```python
from build123d import *

# Parameters (mm, degrees)
SKIZZE1_W                                            = 50
SKIZZE1_H                                            = 60
AUFSATZ_LINEAR_AUSTRAGEN1_DEPTH                      = 5
FORMSENKUNG_F_R_M5_LINSENSENKSCHRAUBE_MI_D           = 5.5
FORMSENKUNG_F_R_M5_LINSENSENKSCHRAUBE_MI_DEPTH       = 20
FORMSENKUNG_F_R_M5_LINSENSENKSCHRAUBE_MI_CSINK_D     = 11
FORMSENKUNG_F_R_M5_LINSENSENKSCHRAUBE_MI_CSINK_ANGLE = 90
FORMSENKUNG_F_R_M5_LINSENSENKSCHRAUBE_MI_TIP         = 1.652366702
KERNLOCH_F_R_M4_GEWINDE1_D                           = 3.3
KERNLOCH_F_R_M5_GEWINDE1_D                           = 4.2
VERRUNDUNG1_R                                        = 3


with BuildPart() as part:
    # Skizze1 → Aufsatz-Linear austragen1 (new body)
    with BuildSketch(Plane.XY):
        with Locations((0, 30)):
            Rectangle(SKIZZE1_W, SKIZZE1_H)
    extrude(amount=-AUFSATZ_LINEAR_AUSTRAGEN1_DEPTH)

    # Formsenkung für M5 Linsensenkschraube mit Schlitz1
    with Locations(Plane.XY):
        with Locations((-16, 10), (16, 10)):
            CounterSinkHole(FORMSENKUNG_F_R_M5_LINSENSENKSCHRAUBE_MI_D / 2, FORMSENKUNG_F_R_M5_LINSENSENKSCHRAUBE_MI_CSINK_D / 2, depth=FORMSENKUNG_F_R_M5_LINSENSENKSCHRAUBE_MI_DEPTH, counter_sink_angle=FORMSENKUNG_F_R_M5_LINSENSENKSCHRAUBE_MI_CSINK_ANGLE)
            with Locations((0, 0, -(FORMSENKUNG_F_R_M5_LINSENSENKSCHRAUBE_MI_DEPTH + FORMSENKUNG_F_R_M5_LINSENSENKSCHRAUBE_MI_TIP / 2))):  # 118° drill point
                Cone(0, FORMSENKUNG_F_R_M5_LINSENSENKSCHRAUBE_MI_D / 2, FORMSENKUNG_F_R_M5_LINSENSENKSCHRAUBE_MI_TIP, mode=Mode.SUBTRACT)

    # Kernloch für M4 Gewinde1 (through all)
    with Locations(Plane.XY):
        with Locations((-14, 19.75), (14, 19.75), (-14, 49.75), (14, 49.75)):
            Hole(KERNLOCH_F_R_M4_GEWINDE1_D / 2)

    # Kernloch für M5 Gewinde1 (through all)
    with Locations(Plane.XY):
        with Locations((-13, 38), (13, 38)):
            Hole(KERNLOCH_F_R_M5_GEWINDE1_D / 2)

    # Verrundung1
    verrundung1_edges = [part.edges().sort_by_distance(p)[0] for p in [
        (25, 0, -2.5),
        (-25, 0, -2.5),
        (-25, 60, -2.5),
        (25, 60, -2.5),
    ]]
    fillet(verrundung1_edges, radius=VERRUNDUNG1_R)


solid = part.part
```
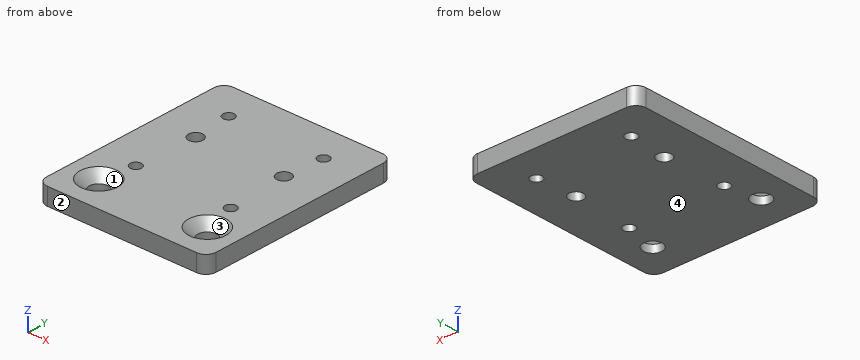
CAD build for the part. Positions are in the model's coordinates, mm. Face numbers are marked on the shaded views. Round coordinates to 2 decimals unless told otherwise and drop trailing zeros. Write each loop counter-clockwise with the first axis right and the second up, starting at its lowest first coordinate (ties: lowest second). Pieces come first, ordered by that corner, then holes.
Item 1: Band-saw the part on A-A on z = -0.9. Give the number of separate pieces and of enclosed holes in the cut face, then the cut area to 3 significant figures.
Filled in:
separate pieces: 1
enclosed holes: 8
area: 2,800 mm2
Item 2: Drop a flat-ended pin along its axis: pin 1 Ø3.5 at (x, y) = (-16, 10) entering from -Z. Give the stop position or say it passes through.
Filled in:
pin 1: passes through
Item 3: Mould opens along Y. For the marked faces 1, 2, 3 and 4 say: released by +Y, released by -Y, zero draft, split by the parting line, or undercut.
Filled in:
face 1: undercut
face 2: released by -Y
face 3: undercut
face 4: zero draft
Item 4: Band-saw the part on B-B on y = 38. Write the cut outline in (x, z), then the cut area to 3 significant figures.
Filled in:
outline: (-25, -5) - (-15.1, -5) - (-15.1, 0) - (-25, 0) - close; (-10.9, -5) - (10.9, -5) - (10.9, 0) - (-10.9, 0) - close; (15.1, -5) - (25, -5) - (25, 0) - (15.1, 0) - close
area: 208 mm2
Item 5: Band-saw the part on C-C on y = 49.75. Write the cut outline in (x, z), then the cut area to 3 significant figures.
Filled in:
outline: (-25, -5) - (-15.65, -5) - (-15.65, 0) - (-25, 0) - close; (-12.35, -5) - (12.35, -5) - (12.35, 0) - (-12.35, 0) - close; (15.65, -5) - (25, -5) - (25, 0) - (15.65, 0) - close
area: 217 mm2
Item 6: Drill centre lines: L1, parallel to X at y = 10, z = -3.55; L2, parallel to Y at x = 14, z = -2.55; L3, parallel to Y at x = -14, z = -2.65. Where is each one in solid material? Low to high.
Filled in:
L1: x = -25 to -18.75, -13.25 to 13.25, 18.75 to 25
L2: y = 0 to 7.83, 12.17 to 18.1, 21.4 to 36.15, 39.85 to 48.1, 51.4 to 60
L3: y = 0 to 7.97, 12.03 to 18.1, 21.4 to 36.15, 39.85 to 48.1, 51.4 to 60
